```python
from build123d import *

# Parameters (mm, degrees)
SKETCH2_W           = 215
SKETCH2_H           = 15
BOSS_EXTRUDE1_DEPTH = 1.6
SKETCH4_W           = 4
SKETCH4_H           = 2.9
BOSS_EXTRUDE2_DEPTH = 2.28


with BuildPart() as part:
    # Sketch2 → Boss-Extrude1 (new body)
    with BuildSketch(Plane(origin=(0, 0, 0), x_dir=(1, 0, 0), z_dir=(0, 1, 0))):
        Rectangle(SKETCH2_W, SKETCH2_H)
    extrude(amount=BOSS_EXTRUDE1_DEPTH)

    # Sketch4 → Boss-Extrude2 (add)
    with BuildSketch(Plane(origin=(0, 1.6, 0), x_dir=(1, 0, 0), z_dir=(0, 1, 0))):
        with Locations((-96.7, -4.2)):
            Rectangle(SKETCH4_W, SKETCH4_H)
        with Locations((-79.118, -4.2)):
            Rectangle(SKETCH4_W, SKETCH4_H)
        with Locations((-61.536, -4.2)):
            Rectangle(SKETCH4_W, SKETCH4_H)
        with Locations((-43.955, -4.2)):
            Rectangle(SKETCH4_W, SKETCH4_H)
        with Locations((-26.373, -4.2)):
            Rectangle(SKETCH4_W, SKETCH4_H)
        with Locations((-8.791, -4.2)):
            Rectangle(SKETCH4_W, SKETCH4_H)
        with Locations((8.791, -4.2)):
            Rectangle(SKETCH4_W, SKETCH4_H)
        with Locations((26.373, -4.2)):
            Rectangle(SKETCH4_W, SKETCH4_H)
        with Locations((43.955, -4.2)):
            Rectangle(SKETCH4_W, SKETCH4_H)
        with Locations((61.536, -4.2)):
            Rectangle(SKETCH4_W, SKETCH4_H)
        with Locations((79.118, -4.2)):
            Rectangle(SKETCH4_W, SKETCH4_H)
        with Locations((96.7, -4.2)):
            Rectangle(SKETCH4_W, SKETCH4_H)
    extrude(amount=BOSS_EXTRUDE2_DEPTH)


solid = part.part
```
Here's how the part is built. I have some questions about the finished solid (model axes, mm). Coordinates: 2 decimals unless noted, no trailing zeros. Loops run counter-clockwise (first coordinate to the right, second up) from the corner with the lowest first, then second, coordinate; pieces in that order, holes last. Notation, with made-up numbers: (-1.5, 31.25) - (23.5, 31.25) arc R24 ccw to (23.5, 61.25) - close; hole circle Ø10 at (-14, 5.5). An arc over 180 degrees is marked (long way). Answer as CSV lines item,"result".
Q1. If I drill on L1, parallel to Y at x = -85, z = -3.25; L2, parallel to Z at x = -24.5, y = 3.55, over which ranges is the centre line in solid material (lowest first)? Write a range as [from, to].
Response:
L1,"[0, 1.6]"
L2,"[2.75, 5.65]"
Q2. For pin 1 (1.8 mm diameter, centred on y = 3, z = 5, fed in from -X); pin 2 (0.7 mm diameter, centred on x = 44, y = 3, fed in from -Z); pin 3 (1.8 mm diameter, centred on x = 45, y = 3, fed in from +Z), each with a flat end and sliding along its axis, tell me the tip position at first contact or that it passes through.
Response:
pin 1,"x = -98.7"
pin 2,"z = 2.75"
pin 3,"z = 5.65"
Q3. If we section it at B-B, the plane z = -0.5: Write out the boundary of the cut face in (x, y).
Response:
outline,"(-107.5, 0) - (107.5, 0) - (107.5, 1.6) - (-107.5, 1.6) - close"
Q4. We'd pull the mould along X, two halves only. Please class faces 1 (the face through (-2, 1.6, 0)), 2 (the face through (-2, 0, 0)): pulls with the +X half, pulls with the -X half, needs draft (parallel to the pull), parting line crosses it, or undercut.
Response:
face 1,"undercut"
face 2,"needs draft"
Q5. If we section it at A-A, the plane x = -79: Write out the boundary of the cut face in (y, z), and give its area (3 significant figures).
Response:
outline,"(0, -7.5) - (1.6, -7.5) - (1.6, 2.75) - (3.88, 2.75) - (3.88, 5.65) - (1.6, 5.65) - (1.6, 7.5) - (0, 7.5) - close"
area,"30.6 mm2"
